```python
from build123d import *

# Parameters (mm, degrees)
ESQUISSE3_W        = 80
ESQUISSE3_H        = 80
BOSS_EXTRU_1_DEPTH = 3


with BuildPart() as part:
    # Esquisse3 → Boss.-Extru.1 (new body)
    with BuildSketch(Plane(origin=(0, 0, 0), x_dir=(1, 0, 0), z_dir=(0, 1, 0))):
        Rectangle(ESQUISSE3_W, ESQUISSE3_H)
    extrude(amount=BOSS_EXTRU_1_DEPTH)

    # Esquisse4 → Révolution1 (revolve)
    with BuildSketch(Plane.XY):
        Polygon((33.000906918, 3), (40, 83), (37, 83), (30.000906918, 3), align=None)
    revolve(axis=Axis((0, 5.327964133, 0), (0, 1, 0)))


solid = part.part
```
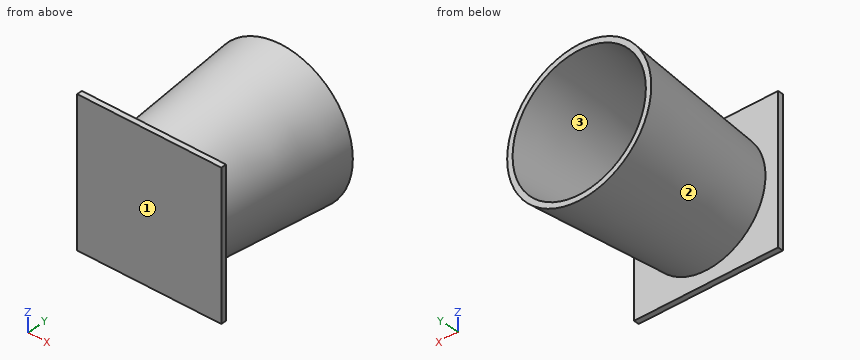
CAD build for the part. Positions are in the model's coordinates, mm. Face numbers are marked on the shaded views. Give positions to 0.01 mm unless a question says otherwise; leave off trailing zeros. Order: outer loops, then holes, each group sorted by start corner. A loop starts at its lowest first (then second) coordinate and runs counter-clockwise, first axis right, second up.
(1) Mould opens along Y. For the marked faces 1, 2 and 3 say: released by +Y, released by -Y, zero draft, split by the parting line, or undercut.
(2) Saw through at B-B, the plane y = 47. Give the cut face in (x, z).
(3) Drill centre lines: L1, parallel to Y at x = 32, z = 27.5; L2, parallel to Z at x = 24.5, y = 59.5; L3, parallel to Z at x = -12, y = 13. Where is each one in solid material? Low to high.
(4) Saw through at D-D, the plane y = 21. Give the cut face in (x, z), then the cut area to 3 significant figures.
(5) Saw through at C-C, the plane z = 0. Give the cut face in (x, y).
(6) Saw through at A-A, the plane x = 0. Give the cut face in (y, z).
(7) Flat gauge pins, fed straight in: pin 1 (6 mm diameter, centred on x = -6, z = 2.5, fed in from +Y); pin 2 (1.5 mm diameter, centred on y = 54, z = -30, fed in from -X); pin 3 (4 mm diameter, centred on x = -27, y = 60, fed in from -Z). Where does each tip first touch, or does it go through?
Results found:
1. face 1: released by -Y
1. face 2: undercut
1. face 3: released by +Y
2. outline: circle Ø73.7 at (0, 0); hole circle Ø67.7 at (0, 0)
3. L1: y = 0 to 3
3. L2: z = -28.97 to -24.92, 24.92 to 28.97
3. L3: z = -31.68 to -28.45, 28.45 to 31.68
4. outline: circle Ø69.15 at (0, 0); hole circle Ø63.15 at (0, 0)
4. area: 623 mm2
5. outline: (-40, 0) - (40, 0) - (40, 3) - (33, 3) - (40, 83) - (37, 83) - (30, 3) - (-30, 3) - (-37, 83) - (-40, 83) - (-33, 3) - (-40, 3) - close
6. outline: (0, -40) - (3, -40) - (3, -33) - (83, -40) - (83, -37) - (3, -30) - (3, 30) - (83, 37) - (83, 40) - (3, 33) - (3, 40) - (0, 40) - close
7. pin 1: stops at y = 3
7. pin 2: stops at x = -23.41
7. pin 3: stops at z = -28.62
